```python
from build123d import *

# Parameters (mm, degrees)
SKETCH2_R                = 20
BOSS_EXTRUDE1_DEPTH      = 45
SKETCH3_R                = 30
BOSS_EXTRUDE2_DEPTH      = 50
BOSS_EXTRUDE3_DEPTH      = 25
BOSS_EXTRUDE3_DEPTH_BACK = 115
SKETCH4_R                = 20
CUT_EXTRUDE1_DEPTH       = 10


with BuildPart() as part:
    # Sketch2 → Boss-Extrude1 (new, symmetric)
    with BuildSketch(Plane.XY):
        with BuildLine():
            Line((-80.985865724, 41), (-80.985865724, -41))
            Line((-80.985865724, -41), (106.905960483, -49.424273902))
            ThreePointArc((106.905960483, -49.424273902), (108.756170043, -49.335499296), (110.558264434, -48.906999406))
            ThreePointArc((110.558264434, -48.906999406), (145.643610678, 0), (110.558264434, 48.906999406))
            ThreePointArc((110.558264434, 48.906999406), (108.756170043, 49.335499296), (106.905960483, 49.424273902))
            Line((106.905960483, 49.424273902), (-80.985865724, 41))
        make_face()
        with Locations(Location((94.014134276, 0, 0), (0, 0, 180))):
            Circle(SKETCH2_R, mode=Mode.SUBTRACT)
    extrude(amount=BOSS_EXTRUDE1_DEPTH, both=True)

    # Sketch3 → Boss-Extrude2 (add)
    with BuildSketch(Plane.ZY.offset(80.985865724)):
        Circle(SKETCH3_R)
    extrude(amount=BOSS_EXTRUDE2_DEPTH)

    # Sketch4 → Boss-Extrude3 (add, two sides: drawn at the far end of the back side and taken through both)
    with BuildSketch(Plane.XY.offset(45).offset(-BOSS_EXTRUDE3_DEPTH_BACK)):
        with Locations((94.014134276, 0)):
            Circle(SKETCH4_R)
    extrude(amount=BOSS_EXTRUDE3_DEPTH + BOSS_EXTRUDE3_DEPTH_BACK)

    # Sketch5 → Cut-Extrude1 (cut)
    with BuildSketch(Plane.XY.offset(45)):
        with BuildLine():
            Line((-61.758305815, 10), (18.241694185, 10))
            ThreePointArc((18.241694185, 10), (28.241694185, 0), (18.241694185, -10))
            Line((18.241694185, -10), (-61.758305815, -10))
            ThreePointArc((-61.758305815, -10), (-71.758305815, 0), (-61.758305815, 10))
        make_face()
    cut_extrude1 = extrude(amount=-CUT_EXTRUDE1_DEPTH, mode=Mode.SUBTRACT)

    # Mirror1: Cut-Extrude1 across plane
    add(cut_extrude1.mirror(Plane.XY), mode=Mode.SUBTRACT)


solid = part.part
```
Geometry check sheet. Reference: the model listing, model coordinates, mm. A direction names the side the tool comes from. Coordinates: 2 decimals unless noted, no trailing zeros. Write each loop counter-clockwise with the first axis right and the second up, starting at its lowest first coordinate (ties: lowest second). Pieces come first, ordered by that corner, then holes. Notation, with made-up numbers: M 12,78.25 L 71,78.25 A14 ccw 71,104.25 Z; hole C 67,8 d8. An arc over 180 degrees is marked long. Use one line per item in the form item = value. Start each with the question number.
1) Section check C-C on x = -3. Enter the section's corners in (y, z), and give its area (3 significant figures).
2) Set-up check for faces 4 (the flat face through (94, 0, -70)), 5 (the flat face through (-80.986, 1, 31)), 6 (the flat face through (11.645, -45.153, 0.63)), 7 (the cylindrical face through (28.24, 0.22, 40.07)), 8 (the cylindrical face through (74.033, 0.879, -57.675)): record each of +Z, -Z, +X, -X, +Y, -Y from which the full face is reachable in a straight line by a thin tool's end or side.
3) Go/stop test with flat-tipped pins: pin 1 Ø8 at (x, z) = (-22.5, -41) entering from +Y; pin 2 Ø8 at (x, z) = (-3, 40) entering from -Y; pin 3 Ø8 at (x, y) = (67, 36) entering from -Z. Record where each tip stops, or that it passes through.
4) Thickness scan on probe 1 along Z at (x, y) = (113, -16); probe 2 along Z at (x, y) = (-40.5, -0.5); probe 3 along Y at (x, z) = (6.5, 37.5). Record the ranges inside material, lowest first. Write a range as from..to.
5) Release check for a two-part mould opening along X. For faces 1 (the flat face through (14.28, 45.27, 0.63)), 2 (the flat face through (-21, -10, -40)), 3 (the flat face through (31, 1, 45)) record: pulls with the +X half, pulls with the -X half, needs draft (parallel to the pull), parting line crosses it, or undercut.
6) Section check A-A on z = 0. Enter the section's corners in (x, y).
7) Section check D-D on z = -50.5. Enter the section's corners in (x, y).
8) Section check B-B on y = 0. Enter the section's corners in (x, z), and give its area (3 significant figures).
Responses:
q1.outline = M -44.5,-45 L -10,-45 L -10,-35 L 10,-35 L 10,-45 L 44.5,-45 L 44.5,45 L 10,45 L 10,35 L -10,35 L -10,45 L -44.5,45 Z
q1.area = 7,610 mm2
q2.face_4 = -Z, +X, -X, +Y, -Y
q2.face_5 = -X
q2.face_6 = +Z, -Z, -X, -Y
q2.face_7 = +Z
q2.face_8 = -Z
q3.pin_1 = 43.8
q3.pin_2 = -44.68
q3.pin_3 = -45
q4.probe_1 = -45..45
q4.probe_2 = -35..35
q4.probe_3 = -44.92..-10, 10..44.92
q5.face_1 = pulls with the -X half
q5.face_2 = undercut
q5.face_3 = needs draft
q6.outline = M -130.99,-30 L -80.99,-30 L -80.99,-41 L 106.91,-49.42 A10 ccw 110.56,-48.91 A51.63 ccw 110.56,48.91 A10 ccw 106.91,49.42 L -80.99,41 L -80.99,30 L -130.99,30 Z
q7.outline = C 94.01,0 d40
q8.outline = M -130.99,-30 L -80.99,-30 L -80.99,-45 L -71.76,-45 L -71.76,-35 L 28.24,-35 L 28.24,-45 L 74.01,-45 L 74.01,-70 L 114.01,-70 L 114.01,-45 L 145.64,-45 L 145.64,45 L 114.01,45 L 114.01,70 L 74.01,70 L 74.01,45 L 28.24,45 L 28.24,35 L -71.76,35 L -71.76,45 L -80.99,45 L -80.99,30 L -130.99,30 Z
q8.area = 23,400 mm2
